Autodesk Inventor part; units mm, degrees
ref_plane "WorkPlane1" through (0, 0, 0) normal (0, 0, 1) x (1, 0, 0)
ref_plane "Work Plane2" through (0, 0, -1.6) normal (0, 0, 1) x (1, 0, 0)
ref_plane "WorkPlane2" through (0, 0, 1) normal (0, 0, 1) x (1, 0, 0)
ref_plane "WorkPlane1" through (0, 0, 0) normal (0, 0, 1) x (1, 0, 0)
ref_plane "Work Plane2" through (0, 0, -1.6) normal (0, 0, 1) x (1, 0, 0)
ref_plane "WorkPlane2" through (0, 0, 1) normal (0, 0, 1) x (1, 0, 0)
sketch "Sketch1" plane through (0, 0, 0) normal (0, 0, 1) x (1, 0, 0)
  point P0 (0, 0)
sketch "Sketch2" plane through (0, 0, 0) normal (0, 0, 1) x (1, 0, 0)
  line L0 (6.5, -19.1956) -> (5.6764, -16.6388)
  arc A0 (9.1452, -14.132) -> (5.6764, -16.6388) centre (7.818, -15.9489) ccw
  line L1 (9.1452, -14.132) -> (10.9421, -15.4445)
  arc A1 (10.9421, -15.4445) -> (-10.9421, -15.4445) centre (0, 0) ccw
  line L2 (-9.1452, -14.132) -> (-10.9421, -15.4445)
  arc A2 (-5.6764, -16.6388) -> (-9.1452, -14.132) centre (-7.818, -15.9489) ccw
  line L3 (-6.5, -19.1956) -> (-5.6764, -16.6388)
  arc A3 (6.5, -19.1956) -> (-6.5, -19.1956) centre (0, 0.9833) ccw
  line L4 (0, 0.9833) -> (-6.5, -19.1956) construction
  line L5 (0, 0.9833) -> (6.5, -19.1956) construction
  dimension "d2" = 21.2
  dimension "d4" = 0
  dimension "d6" = 18.9278
  dimension "d8" = 0.9833
  dimension "d10" = 6.5
  dimension "d12" = 6.5
  dimension "d14" = 2.25
  dimension "d16" = 2.25
  dimension "d18" = 18.65
  dimension "d20" = 18.65
  dimension "d22" = 36
  dimension "d24" = 36
extrude "Extrusion1" add sketch "Sketch2" along normal blind 1.6
sketch "Sketch3" plane through (0, 0, 1.6) normal (0, 0, 1) x (1, 0, 0)
  arc A0 (-5.6764, -16.6388) -> (-9.1452, -14.132) centre (-7.818, -15.9489) ccw
hole "Hole1" at (-7.818, -15.9489, 1.6) direction (0, 0, -1) diameter 2.5 end through all
sketch "Sketch4" plane through (0, 0, 1.6) normal (0, 0, 1) x (1, 0, 0)
  arc A0 (9.1452, -14.132) -> (5.6764, -16.6388) centre (7.818, -15.9489) ccw
hole "Hole2" at (7.818, -15.9489, 1.6) direction (0, 0, -1) diameter 2.5 end through all
equation "\"d29\" = Diam5"
equation "\"d36\" = Diam5"
equation "\"d2\" = 0.5 * Diam2"
equation "\"d6\" = 0.5 * msp_dd1"
equation "\"d8\" = -0.5 * msp_dd1 + 0.5 * Diam2 - 0.222222 * ParA"
equation "\"d10\" = 2.6 * Diam5"
equation "\"d12\" = 2.6 * Diam5"
equation "\"d14\" = 0.9 * Diam5"
equation "\"d16\" = 0.9 * Diam5"
equation "\"d18\" = 1.3 * Diam5 + 0.5 * Diam2 - ParA"
equation "\"d20\" = 1.3 * Diam5 + 0.5 * Diam2 - ParA"
equation "\"d25\" = ParS"
equation "\"Diam5\" = 2.5"
equation "\"ParA\" = 5.8"
equation "\"ParS\" = 1.6"
equation "\"Diam2\" = 42.4"
equation "\"msp_dd1\" = -b + Diam2 - 0.111111 * ParA"
equation "\"msp_pom\" = 0.5 * Diam2 - b"
equation "\"TEMPLATE\" = 1.2345"
properties part number "Кольцо стопорное внутреннее" material "Steel, Mild"
Could you check a few things on this model? Use its own coordinates, in mm. A direction names the side the tool comes from. Give positions to 0.01 mm unless a question says otherwise; leave off trailing zeros. Order: outer loops, then holes, each group sorted by start corner. A loop starts at its lowest first (then second) coordinate and runs counter-clockwise, first axis right, second up. Notation, with made-up numbers: (14.5, 67.25) - (45.5, 67.25) arc R29 ccw to (45.5, 102.25) - close; hole circle Ø10 at (-15, 60). An arc over 180 degrees is marked (long way). Return JSON: item names as keys, results as strings. Group by question number.
Q1. Suppose I cut it at B-B, the plane x = -14.5. Please give me the cut outline in (y, z).
Q2. Which directions (+Z, -Z, +X, -X, +Y, -Y) give clear straight access to the entire face, cutting with the end or side of a thin tool? Please do faces 1 (the face through (6.094, -17.935, 0.789)), 2 (the face through (10.03, -14.78, 0.79)), 3 (the face through (-10, 17, 0)).
Q3. Suppose I cut it at A-A, the plane y = 0. Please give me the cut outline in (x, z).
Q4. Please list where these lines run through material, in increasing order: line 1 along X through (y, z) = (-16.5, 0.3); line 2 along Y through (x, z) = (8.5, 1.3); line 3 along X through (y, z) = (-4.5, 1.3). Write a range as [from, to].
Q5. Suppose I cut it at C-C, the plane y = -16. Please give me the cut outline in (x, z).
Q6. Suppose I cut it at D-D, the plane z = 1.05. Please give me the cut outline in (x, y).
Q7. Thinking about a two-plate mould opening in Y: for faces 4 (the face through (-10.03, -14.78, 0.79)), 5 (the face through (-6.094, -17.935, 0.789)), 6 (the face through (-10, 17, 1.6)), which applies, pulls with the +Y half, pulls with the -Y half, needs draft (parallel to the pull), parting line crosses it, or undercut?
Resolved:
{
 "1": {"outline": "(-14.48, 0) - (-12.17, 0) - (-12.17, 1.6) - (-14.48, 1.6) - close; (12.17, 0) - (16.45, 0) - (16.45, 1.6) - (12.17, 1.6) - close"},
 "2": {"face 1": "+Z, -Z, -Y", "face 2": "+Z, -Z", "face 3": "-Z, +X, -X, +Y, -Y"},
 "3": {"outline": "(-21.18, 0) - (-18.93, 0) - (-18.93, 1.6) - (-21.18, 1.6) - close; (18.93, 0) - (21.18, 0) - (21.18, 1.6) - (18.93, 1.6) - close"},
 "4": {"line 1": "x = [-11.99, -8.94], [-6.7, -5.64], [5.64, 6.7], [8.94, 11.99]", "line 2": "y = [-18.44, -17], [-14.9, -13.8], [16.91, 20.4]", "line 3": "x = [-20.48, -18.39], [18.39, 20.48]"},
 "5": {"outline": "(-12.69, 0) - (-9.07, 0) - (-9.07, 1.6) - (-12.69, 1.6) - close; (-6.57, 0) - (-5.57, 0) - (-5.57, 1.6) - (-6.57, 1.6) - close; (5.57, 0) - (6.57, 0) - (6.57, 1.6) - (5.57, 1.6) - close; (9.07, 0) - (12.69, 0) - (12.69, 1.6) - (9.07, 1.6) - close"},
 "6": {"outline": "(-10.94, -15.44) arc R18.93 cw (long way) to (10.94, -15.44) - (9.15, -14.13) arc R2.25 ccw to (5.68, -16.64) - (6.5, -19.2) arc R21.2 ccw (long way) to (-6.5, -19.2) - (-5.68, -16.64) arc R2.25 ccw to (-9.15, -14.13) - close; hole circle Ø2.5 at (-7.82, -15.95); hole circle Ø2.5 at (7.82, -15.95)"},
 "7": {"face 4": "undercut", "face 5": "pulls with the -Y half", "face 6": "needs draft"}
}
